```python
from build123d import *

# Parameters (mm, degrees)
SKETCH3_W           = 63.5
SKETCH3_H           = 76.2
BOSS_EXTRUDE1_DEPTH = 63.5
SKETCH20_W          = 57.288750963
SKETCH20_H          = 51.688361778
CUT_EXTRUDE2_DEPTH  = 106.747278632
SKETCH21_R          = 12.7
CUT_EXTRUDE4_DEPTH  = 6.063211567


with BuildPart() as part:
    # Sketch3 → Boss-Extrude1 (new body)
    with BuildSketch(Plane(origin=(0, 0, 0), x_dir=(0, 0, -1), z_dir=(1, 0, 0))):
        with Locations((-4.90783597, -0.71667611)):
            Rectangle(SKETCH3_W, SKETCH3_H)
    extrude(amount=BOSS_EXTRUDE1_DEPTH)

    # Sketch20 → Cut-Extrude2 (cut, through all)
    with BuildSketch(Plane(origin=(0, -38.81667611, 0), x_dir=(-1, 0, 0), z_dir=(0, -1, 0))):
        with Locations((-28.644375482, -4.750443514)):
            Rectangle(SKETCH20_W, SKETCH20_H)
    extrude(amount=-CUT_EXTRUDE2_DEPTH, mode=Mode.SUBTRACT)

    # Sketch21 → Cut-Extrude4 (cut)
    with BuildSketch(Plane.XY.offset(36.65783597)):
        with Locations((31.75, -0.71667611)):
            Circle(SKETCH21_R)
    extrude(amount=-CUT_EXTRUDE4_DEPTH, mode=Mode.SUBTRACT)


solid = part.part
```
Check sheet for the modelled part. Datum: model origin and axes. Units: mm. A direction names the side the tool comes from. Round coordinates to 2 decimals unless told otherwise and drop trailing zeros. Order: outer loops, then holes, each group sorted by start corner. A loop starts at its lowest first (then second) coordinate and runs counter-clockwise, first axis right, second up.
1) Section check D-D (z = 7). Record the boundary of the cut face in (x, y), and give its area (3 significant figures).
2) Tool access check on faces 1 (the flat face through (29, -1, -21.094)), 2 (the cylindrical face through (43.864, 3.098, 33.669)), 3 (the flat face through (0, 0, 34)). Record the directions out of +Z, -Z, +X, -X, +Y, -Y that give a thin tool (end or side, any length) a straight path to the whole face; none if there is none.
3) Section check B-B (x = 31.75). Record the boundary of the cut face in (y, z), and give its area (3 significant figures).
4) Scan lines: line 1 (Z direction, x = 10, y = -12.5); line 2 (Y direction, x = 31.75, z = 34.5); line 3 (X direction, y = 30, z = 15.5). Record each from-to range of solid material in increasing order.
5) Section check C-C (y = 30). Record the boundary of the cut face in (x, z), and give its area (3 significant figures).
6) Mould release check, pull along Z, two halves, no side actions. Record for faces 4 (the flat face through (16, -1, 30.595)), 5 (the flat face through (31, -1, -26.842)), 6 (the flat face through (45, -1, 36.658)), 7 (the flat face through (57.5, 37.383, 7.4)): +Z half, -Z half, draft (parallel to the pull), parting line (faces both ways), or undercut.
7) Go/stop test with flat-tipped pins: pin 1 Ø4 at (x, y) = (27.5, -9) entering from +Z; pin 2 Ø4 at (y, z) = (10.5, 0) entering from -X. Record where each tip stops, or that it passes through.
8) Section check A-A (x = 50). Record the boundary of the cut face in (y, z), and give its area (3 significant figures).
Result:
1. outline: (57.29, -38.82) - (63.5, -38.82) - (63.5, 37.38) - (57.29, 37.38) - close
1. area: 473 mm2
2. face 1: -X, +Y, -Y
2. face 2: +Z
2. face 3: +Z, -Z, -X, +Y, -Y
3. outline: (-38.82, -26.84) - (37.38, -26.84) - (37.38, -21.09) - (-38.82, -21.09) - close; (-38.82, 30.59) - (-13.42, 30.59) - (-13.42, 36.66) - (-38.82, 36.66) - close; (11.98, 30.59) - (37.38, 30.59) - (37.38, 36.66) - (11.98, 36.66) - close
3. area: 746 mm2
4. line 1: z = -26.84 to -21.09, 30.59 to 36.66
4. line 2: y = -38.82 to -13.42, 11.98 to 37.38
4. line 3: x = 57.29 to 63.5
5. outline: (0, -26.84) - (63.5, -26.84) - (63.5, 36.66) - (0, 36.66) - (0, 30.59) - (57.29, 30.59) - (57.29, -21.09) - (0, -21.09) - close
5. area: 1,070 mm2
6. face 4: undercut
6. face 5: -Z half
6. face 6: +Z half
6. face 7: draft
7. pin 1: stops at z = -21.09
7. pin 2: stops at x = 57.29
8. outline: (-38.82, -26.84) - (37.38, -26.84) - (37.38, -21.09) - (-38.82, -21.09) - close; (-38.82, 30.59) - (37.38, 30.59) - (37.38, 36.66) - (-38.82, 36.66) - close
8. area: 900 mm2
